Check sheet for the modelled part. Datum: model origin and axes. Units: mm. A direction names the side the tool comes from. Coordinates: 2 decimals unless noted, no trailing zeros. Loops run counter-clockwise (first coordinate to the right, second up) from the corner with the lowest first, then second, coordinate; pieces in that order, holes last.
```python
from build123d import *

# Parameters (mm, degrees)
F0_R     = 11
F1_DEPTH = 7
F2_R     = 1.75


with BuildPart() as f1:
    # F0 (on Top) → F1 (new body)
    with BuildSketch(Plane.XY):
        Polygon((15, -25.9807621135), (7.5, -12.9903810568), (-7.5, -12.9903810568), (-15, -25.9807621135), (-7.5, -38.9711431703), (7.5, -38.9711431703), align=None)
        with Locations((0, -25.9807621135)):
            Circle(F0_R, mode=Mode.SUBTRACT)
        Polygon((-7.5, -12.9903810568), (7.5, -12.9903810568), (15, 0), (7.5, 12.9903810568), (-7.5, 12.9903810568), (-15, 0), align=None)
        Circle(F0_R, mode=Mode.SUBTRACT)
        Polygon((7.5, 12.9903810568), (15, 0), (30, 0), (37.5, 12.9903810568), (30, 25.9807621135), (15, 25.9807621135), align=None)
        with Locations((22.5, 12.9903810568)):
            Circle(F0_R, mode=Mode.SUBTRACT)
        Polygon((-30, 0), (-15, 0), (-7.5, 12.9903810568), (-15, 25.9807621135), (-30, 25.9807621135), (-37.5, 12.9903810568), align=None)
        with Locations((-22.5, 12.9903810568)):
            Circle(F0_R, mode=Mode.SUBTRACT)
    extrude(amount=F1_DEPTH)

    # F2
    f2_edges = [f1.edges().sort_by_distance(p)[0] for p in [
        (7.5, -38.971143, 3.5),
        (15, -25.980762, 3.5),
        (11.25, -32.475953, 0),
        (11.25, -32.475953, 7),
        (0, -38.971143, 7),
        (11.25, -19.485572, 7),
        (11.25, -19.485572, 0),
        (11.25, -6.495191, 0),
        (7.5, -12.990381, 3.5),
        (11.25, -6.495191, 7),
        (15, 0, 3.5),
        (22.5, 0, 0),
        (22.5, 0, 7),
        (30, 0, 3.5),
        (33.75, 6.495191, 0),
        (33.75, 6.495191, 7),
        (33.75, 19.485572, 0),
        (33.75, 19.485572, 7),
        (37.5, 12.990381, 3.5),
        (30, 25.980762, 3.5),
        (22.5, 25.980762, 7),
        (22.5, 25.980762, 0),
        (11.25, 19.485572, 7),
        (11.25, 19.485572, 0),
        (0, 12.990381, 7),
        (0, 12.990381, 0),
        (-11.25, 19.485572, 7),
        (-11.25, 19.485572, 0),
        (-22.5, 25.980762, 0),
        (-15, 25.980762, 3.5),
        (-22.5, 25.980762, 7),
        (-30, 25.980762, 3.5),
        (-33.75, 19.485572, 7),
        (-33.75, 19.485572, 0),
        (-37.5, 12.990381, 3.5),
        (-33.75, 6.495191, 7),
        (-33.75, 6.495191, 0),
        (-22.5, 0, 0),
        (-30, 0, 3.5),
        (-22.5, 0, 7),
        (-15, 0, 3.5),
        (-11.25, -6.495191, 7),
        (-7.5, -12.990381, 3.5),
        (-11.25, -19.485572, 0),
        (-11.25, -19.485572, 7),
        (-15, -25.980762, 3.5),
        (-11.25, -32.475953, 7),
        (-11.25, -32.475953, 0),
        (-7.5, -38.971143, 3.5),
        (0, -38.971143, 0),
        (-7.5, 12.990381, 3.5),
        (7.5, 12.990381, 3.5),
        (15, 25.980762, 3.5),
        (-11.25, -6.495191, 0),
    ]]
    fillet(f2_edges, radius=F2_R)


solid = f1.part
```
1) Scan lines: line 1 (Y direction, x = 0, z = 4.75); line 2 (X direction, y = 23, z = 4.5); line 3 (Y direction, x = -22.5, z = 2). Record each from-to range of solid material in increasing order.
Answer sheet:
line 1: y = -38.97 to -36.98, -14.98 to -11, 11 to 12.99
line 2: x = -31.72 to -27.06, -17.94 to -13.28, 13.28 to 17.94, 27.06 to 31.72
line 3: y = 0 to 1.99, 23.99 to 25.98
2) Mould release check, pull along X, two halves, no side actions. Record for faces 1 (the cylindrical face through (11.637, 19.157, 0.526)), 2 (the cylindrical face through (33.272, 19.315, 0.526)), 3 (the cylindrical face through (-7.77, -13, 3.52)): +X half, -X half, draft (parallel to the pull), parting line (faces both ways), or undercut.
Answer sheet:
face 1: undercut
face 2: +X half
face 3: -X half
3) Depth check by flat-ended pin: pin 1 (3 mm diameter, centred on x = 19.5, z = 3.5, fed in from -Y); pin 2 (4 mm diameter, centred on x = 3, z = 3, fed in from +Y); pin 3 (8 mm diameter, centred on x = 1, y = 12, fed in from +Z); pin 4 (2 mm diameter, centred on y = -22, z = 6, fed in from -X). Enter the tip coordinate at first touch or a pass-through.
Answer sheet:
pin 1: stops at y = 0
pin 2: stops at y = 12.99
pin 3: stops at z = 7
pin 4: stops at x = -13.19
4) Section check C-C on z = 4. Give the number of separate pieces and of enclosed holes in the cut face, plus the area to 3 significant figures.
Answer sheet:
separate pieces: 1
enclosed holes: 4
area: 817 mm2
5) Section check B-B on x = 22.5. Enter the section's corners in (y, z), plus the area to 3 significant figures.
Answer sheet:
outline: (0, 1.75) arc R1.75 ccw to (1.75, 0) - (1.99, 0) - (1.99, 7) - (1.75, 7) arc R1.75 ccw to (0, 5.25) - close; (23.99, 0) - (24.23, 0) arc R1.75 ccw to (25.98, 1.75) - (25.98, 5.25) arc R1.75 ccw to (24.23, 7) - (23.99, 7) - close
area: 25.2 mm2
6) Set-up check for faces 4 (the cylindrical face through (-22.409, 0.499, 0.526)), 5 (the flat face through (-11.295, -6.417, 3.476)), 6 (the cylindrical face through (7.376, 13.231, 3.524)), 7 (the cylindrical face through (-10.863, -19.814, 6.474)): record each of +Z, -Z, +X, -X, +Y, -Y from which the full face is reachable in a straight line by a thin tool's end or side.
Answer sheet:
face 4: -Z, -X, -Y
face 5: +Z, -Z, -X
face 6: +Z, -Z, +Y
face 7: +Z, -X
7) Section check A-A on x = 0. Enter the section's corners in (y, z), plus the area to 3 significant figures.
Answer sheet:
outline: (-38.97, 1.75) arc R1.75 ccw to (-37.22, 0) - (-36.98, 0) - (-36.98, 7) - (-37.22, 7) arc R1.75 ccw to (-38.97, 5.25) - close; (-14.98, 0) - (-11, 0) - (-11, 7) - (-14.98, 7) - close; (11, 0) - (11.24, 0) arc R1.75 ccw to (12.99, 1.75) - (12.99, 5.25) arc R1.75 ccw to (11.24, 7) - (11, 7) - close
area: 53.1 mm2
